Check sheet for the modelled part. Datum: model origin and axes. Units: mm. Face numbers are marked on the shaded views. Coordinates: 2 decimals unless noted, no trailing zeros. Loops run counter-clockwise (first coordinate to the right, second up) from the corner with the lowest first, then second, coordinate; pieces in that order, holes last. Notation, with made-up numbers: M 41.25,-15.5 L 71.25,-15.5 A23 cw 71.25,0.5 Z; hole C 89,47 d4. An arc over 180 degrees is marked long. Write each question's results on one line, items separated by ' | '. Start each with the question number.
from build123d import *

# Parameters (mm, degrees)
F0_W        = 194
F0_H        = 64.6
F1_DEPTH    = 2
F2_W        = 184
F2_H        = 54.6
F3_DEPTH    = 0.5
F4_R        = 6.25
F4_W        = 2.5
F4_H        = 13.5
F5_DEPTH    = 25
F6_T1_DEPTH = 16.5427907903
F6_T3_DEPTH = 2.4643962848
F7_DEPTH    = 1.5


# Not quite as in the source:
# - a fillet or chamfer that OpenCascade refuses, or shapes differently, is made with other operations: its cross-section is extruded or revolved along the edge and cut away or added


with BuildPart() as f1:
    # F0 (on Top) → F1 (new body)
    with BuildSketch(Plane.XY):
        Rectangle(F0_W, F0_H)
        Polygon((98, 0), (97, 32.3), (97, -32.3), align=None)
        Polygon((-97, -32.3), (-97, 32.3), (-98, 0), align=None)
    extrude(amount=F1_DEPTH)

    # F2 (on face) → F3 (join)
    with BuildSketch(Plane.XY.offset(2)):
        Rectangle(F2_W, F2_H)
    extrude(amount=F3_DEPTH)

    # F4 (on face) → F5 (cut)
    with BuildSketch(Plane.XY.offset(2.5)):
        Polygon((-10, 20.5), (-82, 20.5), (-82, 6.75), (-79.5, 6.75), (-79.5, -6.75), (-82, -6.75), (-82, -20.5), (-10, -20.5), (-10, -6.75), (-12.5, -6.75), (-12.5, 6.75), (-10, 6.75), align=None)
        with Locations((36.375, 0)):
            Circle(F4_R)
        with Locations((55.625, 0)):
            Circle(F4_R)
        with Locations((-11.25, 0)):
            Rectangle(F4_W, F4_H)
        with Locations((-80.75, 0)):
            Rectangle(F4_W, F4_H)
    extrude(amount=-F5_DEPTH, mode=Mode.SUBTRACT)

    # F6: fillet of radius 3 on 6 edges, made by hand

    # F6_s2 → F6_t1 (cut)
    with BuildSketch(Plane.XY.offset(-7.2713953952)):
        with BuildLine():
            ThreePointArc((97.0900051153, -29.3928347763), (96.1796822102, -31.4538923289), (94.0914418419, -32.3))
            Line((94.0914418419, -32.3), (97, -32.3))
            Line((97, -32.3), (97.0900051153, -29.3928347763))
        make_face()
        with BuildLine():
            ThreePointArc((94.0914418419, 32.3), (96.1796822102, 31.4538923289), (97.0900051153, 29.3928347763))
            Line((97.0900051153, 29.3928347763), (97, 32.3))
            Line((97, 32.3), (94.0914418419, 32.3))
        make_face()
        with BuildLine():
            ThreePointArc((-94.0914418419, 32.3), (-96.1796822102, 31.4538923289), (-97.0900051153, 29.3928347763))
            Line((-97.0900051153, 29.3928347763), (-97, 32.3))
            Line((-97, 32.3), (-94.0914418419, 32.3))
        make_face()
        with BuildLine():
            ThreePointArc((-97.0900051153, -29.3928347763), (-96.1796822102, -31.4538923289), (-94.0914418419, -32.3))
            Line((-94.0914418419, -32.3), (-97, -32.3))
            Line((-97, -32.3), (-97.0900051153, -29.3928347763))
        make_face()
    extrude(amount=F6_T1_DEPTH, mode=Mode.SUBTRACT)

    # F6_s4 → F6_t3 (cut)
    with BuildSketch(Plane.XY.offset(-0.2321981424)):
        with BuildLine():
            ThreePointArc((-97.9971258583, 0.0928347763), (-97.998562585, 0), (-97.9971258583, -0.0928347763))
            Line((-97.9971258583, -0.0928347763), (-98, 0))
            Line((-98, 0), (-97.9971258583, 0.0928347763))
        make_face()
        with BuildLine():
            ThreePointArc((97.9971258583, 0.0928347763), (97.998562585, 0), (97.9971258583, -0.0928347763))
            Line((97.9971258583, -0.0928347763), (98, 0))
            Line((98, 0), (97.9971258583, 0.0928347763))
        make_face()
    extrude(amount=F6_T3_DEPTH, mode=Mode.SUBTRACT)

    # F4 (on face) → F7 (cut)
    with BuildSketch(Plane.XY.offset(2.5)):
        Polygon((-10, 20.5), (-82, 20.5), (-82, 6.75), (-79.5, 6.75), (-79.5, -6.75), (-82, -6.75), (-82, -20.5), (-10, -20.5), (-10, -6.75), (-12.5, -6.75), (-12.5, 6.75), (-10, 6.75), align=None)
        with Locations((-80.75, 0)):
            Rectangle(F4_W, F4_H)
        with Locations((-83.25, 0)):
            Rectangle(F4_W, F4_H)
        with Locations((-8.75, 0)):
            Rectangle(F4_W, F4_H)
        with Locations((-11.25, 0)):
            Rectangle(F4_W, F4_H)
        with Locations((36.375, 0)):
            Circle(F4_R)
        with Locations((55.625, 0)):
            Circle(F4_R)
    extrude(amount=-F7_DEPTH, mode=Mode.SUBTRACT)


solid = f1.part
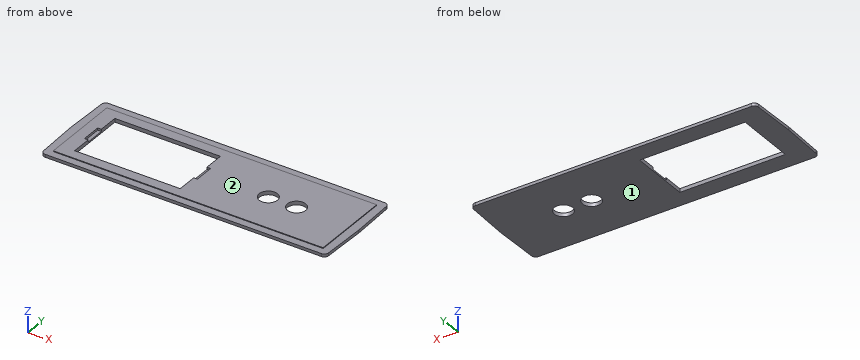
Item 1: Depth check by flat-ended pin: P1, Ø1.5, axis at x = 26.5, y = 0.5, coming from the -Z side; P2, Ø1.5, axis at y = -2.5, z = 1.5, coming from the -X side. Enter the tip coordinate at first touch or a pass-through.
Item 2: Section check A-A (x = -46). Record the cut outline in (y, z), plus the area to 3 significant figures.
Item 3: Section check B-B (z = 0.4). Record the cut outline in (x, y) (3 decimals), plus the area to 3 significant figures.
Item 4: Release check for a two-part mould opening along Z. For the marked faces 1 and 2 record: +Z half, -Z half, draft (parallel to the pull), parting line (faces both ways), or undercut.
Item 5: Thickness scan on line 1 (X direction, y = -11.5, z = 2.2); line 2 (Y direction, x = -41.5, z = 1.9); line 3 (X direction, y = 5, z = 0.2) (3 decimals). Record the ranges inside material, lowest first.
Item 6: Section check D-D (x = 14.5). Record the cut outline in (y, z), plus the area to 4 significant figures.
Item 7: Section check C-C (y = 12). Record the cut outline in (x, z), plus the area to 3 significant figures.
Computed values:
1) P1: stops at z = 0 | P2: stops at x = -97.95
2) outline: M -32.3,0 L -20.5,0 L -20.5,2.5 L -27.3,2.5 L -27.3,2 L -32.3,2 Z; M 20.5,0 L 32.3,0 L 32.3,2 L 27.3,2 L 27.3,2.5 L 20.5,2.5 Z | area: 54.0 mm²
3) outline: M -97.997,-0.093 L -97.09,-29.393 A3 ccw -94.091,-32.3 L 94.091,-32.3 A3 ccw 97.09,-29.393 L 97.997,-0.093 A3 ccw 97.997,0.093 L 97.09,29.393 A3 ccw 94.091,32.3 L -94.091,32.3 A3 ccw -97.09,29.393 L -97.997,0.093 A3 ccw Z; hole M -82,-20.5 L -10,-20.5 L -10,20.5 L -82,20.5 Z; hole C 36.375,0 d12.5; hole C 55.625,0 d12.5 | area: 9,390 mm²
4) face 1: -Z half | face 2: +Z half
5) line 1: x = -92 to -82, -10 to 92 | line 2: y = -32.3 to -20.5, 20.5 to 32.3 | line 3: x = -97.845 to -82, -10 to 32.625, 40.125 to 51.875, 59.375 to 97.845
6) outline: M -32.3,0 L 32.3,0 L 32.3,2 L 27.3,2 L 27.3,2.5 L -27.3,2.5 L -27.3,2 L -32.3,2 Z | area: 156.5 mm²
7) outline: M -97.63,0 L -82,0 L -82,2.5 L -92,2.5 L -92,2 L -97.63,2 Z; M -10,0 L 97.63,0 L 97.63,2 L 92,2 L 92,2.5 L -10,2.5 Z | area: 303 mm²
